Can you work these out from the model? Positions are in its coordinate system, mm. Coordinates: 2 decimals unless noted, no trailing zeros. Order: outer loops, then holes, each group sorted by start corner. A loop starts at its lowest first (then second) coordinate and runs counter-clockwise, first axis right, second up. Notation, with made-up numbers: (-22, 8) -> (24, 8) arc R21 ccw to (24, 42) -> close; hole circle Ø2 at (29.25, 60). An arc over 180 degrees is marked (long way). Answer in a Markdown table with one row per item. Add a question column.
1. Will these pins go through, and if not, where does the flat tip stop? pin 1 (3.5 mm diameter, centred on y = 120, z = -11.72, fed in from +X); pin 2 (2 mm diameter, centred on x = 3, y = 388, fed in from -Z); pin 3 (2 mm diameter, centred on x = 2, y = 453.5, fed in from -Z); pin 4 (1.2 mm diameter, centred on x = 1.5, y = 509.5, fed in from -Z).
2. Imagine slicing it at D-D on z = -76. Write out the boundary of the cut face in (x, y).
3. Imagine slicing it at B-B on z = -145. Write out the boundary of the cut face in (x, y), plus the area to 3 significant figures.
4. If I drill on line 1 along Y through (x, z) = (1.7, -115); line 2 along Y through (x, z) = (0.95, -51); line 3 along Y through (x, z) = (2.6, -258), over which ranges is the centre line in solid material (lowest first)? Write a range as [from, to].
5. Imagine slicing it at C-C on z = -115. Write out the boundary of the cut face in (x, y), plus the area to 3 significant figures.
6. Imagine slicing it at A-A on y = 402.5. Write out the boundary of the cut face in (x, z), plus the area to 3 significant figures.
from build123d import *

# Parameters (mm, degrees)
EXTRUDE_1_DEPTH    = 533.713673317
SKETCH1_W          = 232
SKETCH1_H          = 320
CUT_EXTRUDE1_DEPTH = 611.987450173
SKETCH2_W          = 35
SKETCH2_H          = 6
CUT_EXTRUDE2_DEPTH = 611.987450173
SKETCH3_R          = 6
CUT_EXTRUDE3_DEPTH = 611.987450173
SKETCH4_R          = 2
CUT_EXTRUDE4_DEPTH = 611.987450173


with BuildPart() as part:
    # Эскиз1 → Вытянуть1 (new body)
    with BuildSketch(Plane(origin=(0, 0, 0), x_dir=(1, 0, 0), z_dir=(0, 1, 0))):
        Polygon((0, 0), (4, 1.764508657), (4, 294.827324918), (0, 297.387590837), align=None)
    extrude(amount=EXTRUDE_1_DEPTH)

    # Sketch1 → Cut-Extrude1 (cut, through all)
    with BuildSketch(Plane.ZY):
        with Locations((-149.055893529, 310.5)):
            Rectangle(SKETCH1_W, SKETCH1_H)
    extrude(amount=-CUT_EXTRUDE1_DEPTH, mode=Mode.SUBTRACT)

    # Sketch2 → Cut-Extrude2 (cut, through all)
    with BuildSketch(Plane.ZY):
        with Locations((-229.887590837, 508.5)):
            Rectangle(SKETCH2_W, SKETCH2_H)
        with Locations((-67.5, 508.5)):
            Rectangle(SKETCH2_W, SKETCH2_H)
    extrude(amount=-CUT_EXTRUDE2_DEPTH, mode=Mode.SUBTRACT)

    # Sketch3 → Cut-Extrude3 (cut, through all)
    with BuildSketch(Plane.ZY):
        with Locations((-182.387590837, 518.713673317)):
            Circle(SKETCH3_R)
        with Locations((-115, 518.713673317)):
            Circle(SKETCH3_R)
        with Locations((-182.387590837, 95.5)):
            Circle(SKETCH3_R)
        with Locations((-115, 95.5)):
            Circle(SKETCH3_R)
    extrude(amount=-CUT_EXTRUDE3_DEPTH, mode=Mode.SUBTRACT)

    # Sketch4 → Cut-Extrude4 (cut, through all)
    with BuildSketch(Plane.ZY):
        with Locations((-286.387590837, 496.713673317)):
            Circle(SKETCH4_R)
        with Locations(Location((-11.724196221, 496.713673317, 0), (0, 0, 180))):
            Circle(SKETCH4_R)
        with Locations((-286.387590837, 120)):
            Circle(SKETCH4_R)
        with Locations(Location((-11.724196221, 120, 0), (0, 0, 180))):
            Circle(SKETCH4_R)
    extrude(amount=-CUT_EXTRUDE4_DEPTH, mode=Mode.SUBTRACT)


solid = part.part
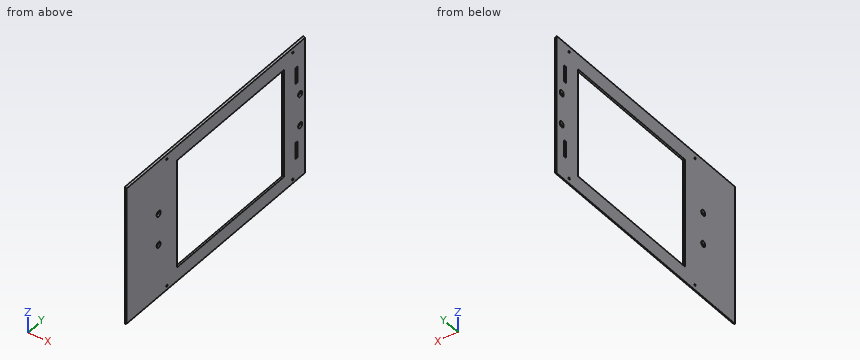
Answers follow:
| question | item | result |
|---|---|---|
| 1 | pin 1 | passes through |
| 1 | pin 2 | stops at z = -296.11 |
| 1 | pin 3 | stops at z = -296.75 |
| 1 | pin 4 | stops at z = -296.81 |
| 2 | outline | (0, 0) -> (4, 0) -> (4, 150.5) -> (0, 150.5) -> close; (0, 470.5) -> (4, 470.5) -> (4, 505.5) -> (0, 505.5) -> close; (0, 511.5) -> (4, 511.5) -> (4, 533.71) -> (0, 533.71) -> close |
| 3 | outline | (0, 0) -> (4, 0) -> (4, 150.5) -> (0, 150.5) -> close; (0, 470.5) -> (4, 470.5) -> (4, 533.71) -> (0, 533.71) -> close |
| 3 | area | 855 mm² |
| 4 | line 1 | y = [0, 89.5], [101.5, 150.5], [470.5, 512.71], [524.71, 533.71] |
| 4 | line 2 | y = [0, 150.5], [470.5, 505.5], [511.5, 533.71] |
| 4 | line 3 | y = [0, 150.5], [470.5, 533.71] |
| 5 | outline | (0, 0) -> (4, 0) -> (4, 89.5) -> (0, 89.5) -> close; (0, 101.5) -> (4, 101.5) -> (4, 150.5) -> (0, 150.5) -> close; (0, 470.5) -> (4, 470.5) -> (4, 512.71) -> (0, 512.71) -> close; (0, 524.71) -> (4, 524.71) -> (4, 533.71) -> (0, 533.71) -> close |
| 5 | area | 759 mm² |
| 6 | outline | (0, -297.39) -> (4, -294.83) -> (4, -265.06) -> (0, -265.06) -> close; (0, -33.06) -> (4, -33.06) -> (4, -1.76) -> (0, 0) -> close |
| 6 | area | 253 mm² |
